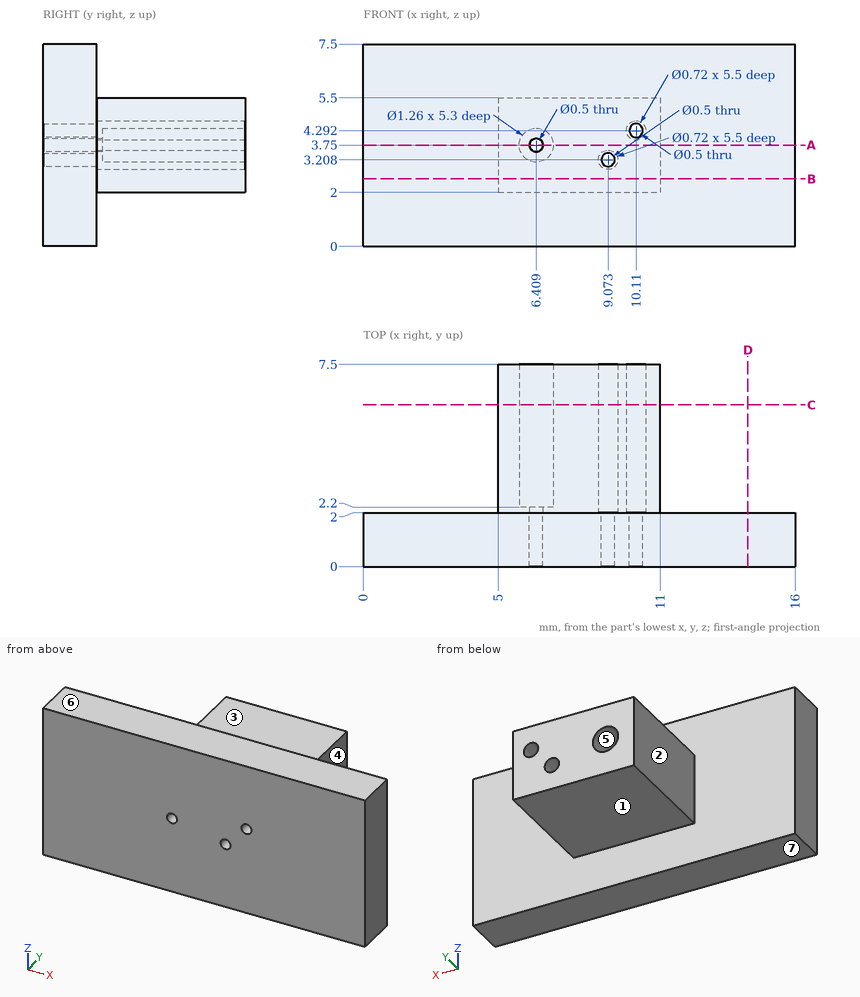
Geometry check sheet. Reference: drawing and pictorial views, mm from the part's lowest x, y, z. A direction names the side the tool comes from. Round coordinates to 2 decimals unless told otherwise and drop trailing zeros. Loops run counter-clockwise (first coordinate to the right, second up) from the corner with the lowest first, then second, coordinate; pieces in that order, holes last. Notation, with made-up numbers: M 37,34.25 L 56,34.25 A27 cw 56,69.25 Z; hole C 22.25,-17.5 d7. An arc over 180 degrees is marked long. Return JSON: item names as keys, results as strings. Group by question number.
(1) Section check D-D, the plane x = 14.25. Enter the section's corners in (y, z).
(2) Scan lines: line 1 along X through (y, z) = (3.5, 3.5) (1 decimal); line 2 along Y through (x, z) = (9, 1.5); line 3 along Z through (x, y) = (7.25, 5.75). Record each from-to range of solid material in increasing order. Write a range as [from, to].
(3) Set-up check for the marked faces 1, 2, 3 and 4: record each of +Z, -Z, +X, -X, +Y, -Y from which the full face is reachable in a straight line by a thin tool's end or side.
(4) Mould release check, pull along Z, two halves, no side actions. Record for the marked faces 5, 6 and 7: pulls with the +Z half, pulls with the -Z half, needs draft (parallel to the pull), parting line crosses it, or undercut.
(5) Go/stop test with flat-tipped pins: pin 1 (4 mm diameter, centred on y = 6, z = 4.5, fed in from -X); pin 2 (4 mm diameter, centred on y = 4.5, z = 4.5, fed in from +X). Record where each tip stops, or that it passes through.
(6) Section check C-C, the plane y = 6. Enter the section's corners in (x, z).
(7) Section check B-B, the plane z = 2.5. Enter the section's corners in (x, y).
(8) Section check A-A, the plane z = 3.75. Enter the section's corners in (x, y).
Data:
{
 "1": {"outline": "M 0,0 L 2,0 L 2,7.5 L 0,7.5 Z"},
 "2": {"line 1": "[5, 5.8], [7, 8.9], [9.3, 11]", "line 2": "[0, 2]", "line 3": "[2, 5.5]"},
 "3": {"face 1": "-Z, +X, -X, +Y", "face 2": "+Z, -Z, -X, +Y", "face 3": "+Z, +X, -X, +Y", "face 4": "+Z, -Z, +X, +Y"},
 "4": {"face 5": "undercut", "face 6": "pulls with the +Z half", "face 7": "pulls with the -Z half"},
 "5": {"pin 1": "x = 5", "pin 2": "x = 11"},
 "6": {"outline": "M 5,2 L 11,2 L 11,5.5 L 5,5.5 Z; hole C 6.41,3.75 d1.26; hole C 9.07,3.21 d0.72; hole C 10.11,4.29 d0.72"},
 "7": {"outline": "M 0,0 L 16,0 L 16,2 L 11,2 L 11,7.5 L 5,7.5 L 5,2 L 0,2 Z"},
 "8": {"outline": "M 0,0 L 6.16,0 L 6.16,2.2 L 5.78,2.2 L 5.78,7.5 L 5,7.5 L 5,2 L 0,2 Z; M 6.66,0 L 16,0 L 16,2 L 11,2 L 11,7.5 L 7.04,7.5 L 7.04,2.2 L 6.66,2.2 Z"}
}
